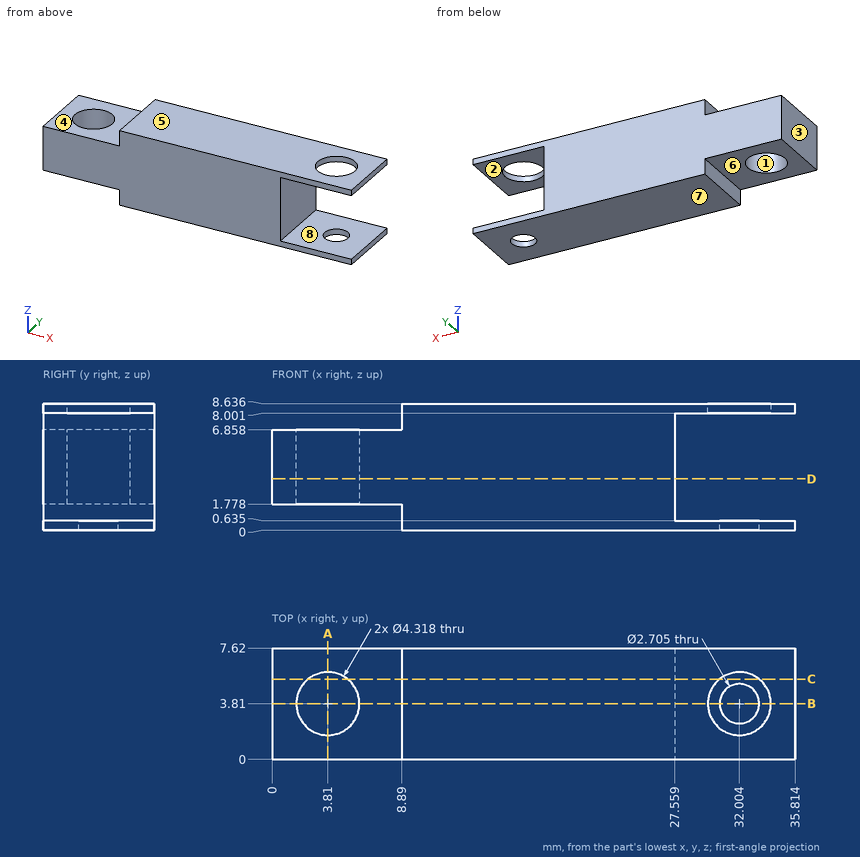
The figure shows three views and two pictorial views of one solid part (mm, origin at its lowest corner). Answer the questions. A direction names the side the tool comes from. Round coordinates to 2 decimals unless told otherwise and drop trailing zeros. Write each loop counter-clockwise with the first axis right and the second up, starting at its lowest first coordinate (ties: lowest second). Pieces come first, ordered by that corner, then holes. Notation, with made-up numbers: (33, 82) - (64, 82) arc R29 ccw to (64, 106) - close; hole circle Ø9 at (22.5, 41.5). An arc over 180 degrees is marked (long way). Use one line per item in the form item = value. Start each with the question number.
Item 1: Find the intervals of material crossed by line 1 (X direction, y = 4, z = 4); line 2 (Z direction, x = 34.5, y = 7.25) (3 decimals); line 3 (Y direction, x = 3.81, z = 4.15), in increasing order. Write a range as [from, to].
Item 2: A tool of negligible diameter and unlimited length cuts with its end or side. For the marked faces 4, 5, 6, 7 and 8, from which of +Z, -Z, +X, -X, +Y, -Y can it reach the whole face along a straight path? Write none if from no direction.
Item 3: Determine the mould class of the marked faces 1, 2 and 3 for opening direction X: +X half, -X half, draft (parallel to the pull), parting line (faces both ways), or undercut.
Item 4: A cutting plane is placed at B-B (y = 3.81). Write down the section's boundary in (x, z) (1 decimal), plus the area to 3 significant figures.
Item 5: A cutting plane is placed at C-C (y = 5.5). Write down the section's boundary in (x, z) (1 decimal).
Item 6: Flat-ended cylindrical pins translate along their axes: pin 1 Ø4 at (x, y) = (4, 4) entering from +Z; pin 2 Ø1.4 at (y, z) = (4, 0.5) entering from -X; pin 3 Ø4 at (x, y) = (4, 3.5) entering from -Z. Find the tip coordinate at first contact, or state that the pin passes through.
Item 7: A cutting plane is placed at D-D (z = 3.5). Write down the section's boundary in (x, y), plus the area to 3 significant figures.
Item 8: A cutting plane is placed at A-A (x = 3.81). Write down the section's boundary in (y, z).
The answers:
q1.line_1 = [0, 1.66], [5.96, 27.56]
q1.line_2 = [0, 0.635], [8.001, 8.636]
q1.line_3 = [0, 1.65], [5.97, 7.62]
q2.face_4 = +Z, -X, +Y, -Y
q2.face_5 = +Z, +X, -X, +Y, -Y
q2.face_6 = -Z, -X, +Y, -Y
q2.face_7 = -Z, +X, -X, +Y, -Y
q2.face_8 = +X, +Y, -Y
q3.face_1 = undercut
q3.face_2 = draft
q3.face_3 = -X half
q4.outline = (0, 1.8) - (1.7, 1.8) - (1.7, 6.9) - (0, 6.9) - close; (6, 1.8) - (8.9, 1.8) - (8.9, 0) - (30.7, 0) - (30.7, 0.6) - (27.6, 0.6) - (27.6, 8) - (29.8, 8) - (29.8, 8.6) - (8.9, 8.6) - (8.9, 6.9) - (6, 6.9) - close; (33.4, 0) - (35.8, 0) - (35.8, 0.6) - (33.4, 0.6) - close; (34.2, 8) - (35.8, 8) - (35.8, 8.6) - (34.2, 8.6) - close
q4.area = 190 mm^2
q5.outline = (0, 1.8) - (2.5, 1.8) - (2.5, 6.9) - (0, 6.9) - close; (5.2, 1.8) - (8.9, 1.8) - (8.9, 0) - (35.8, 0) - (35.8, 0.6) - (27.6, 0.6) - (27.6, 8) - (30.7, 8) - (30.7, 8.6) - (8.9, 8.6) - (8.9, 6.9) - (5.2, 6.9) - close; (33.3, 8) - (35.8, 8) - (35.8, 8.6) - (33.3, 8.6) - close
q6.pin_1 = 6.86
q6.pin_2 = 8.89
q6.pin_3 = 1.78
q7.outline = (0, 0) - (27.56, 0) - (27.56, 7.62) - (0, 7.62) - close; hole circle Ø4.32 at (3.81, 3.81)
q7.area = 195 mm^2
q8.outline = (0, 1.78) - (1.65, 1.78) - (1.65, 6.86) - (0, 6.86) - close; (5.97, 1.78) - (7.62, 1.78) - (7.62, 6.86) - (5.97, 6.86) - close
